The model under review builds one solid part; all positions refer to its coordinate system, in mm. Face numbers are marked on the shaded views. Round coordinates to 2 decimals unless told otherwise and drop trailing zeros. Write each loop counter-clockwise with the first axis right and the second up, starting at its lowest first coordinate (ties: lowest second). Pieces come first, ordered by that corner, then holes.
Item 1: Add section B-B (x = 0). Give the boundary of the cut face in (y, z).
Item 2: Add section A-A (y = 3.75). Give the boundary of the cut face in (x, z), plus the area to 3 significant figures.
Item 3: Clearance check with flat-ended pins moving along their axes: pin 1 Ø3 at (y, z) = (15.5, -5) entering from +X; pin 2 Ø8 at (y, z) = (9, 7.5) entering from -X; pin 3 Ø4 at (x, y) = (13, 3.5) entering from -Z; pin 4 Ø18 at (x, z) = (0, 0) entering from +Y. State where each tip first meets the part, or that it passes through.
Item 4: To check wall thickness, follow L1, parallel to Z at x = 0, y = 7.5; L2, parallel to X at y = 8.5, z = 0; L3, parallel to X at y = 1.25, z = -4. State the ranges of each line that lie inside material, in increasing order.
Item 5: Draft analysis for pull direction Z (two halves, no side actions). For the marked faces 1, 2 and 3, state which applies: +Z half, -Z half, draft (parallel to the pull), parting line (faces both ways), or undercut.
```python
from build123d import *

# Parameters (mm, degrees)
SKETCH5_R           = 10
BOSS_EXTRUDE1_DEPTH = 20


with BuildPart() as part:
    # Sketch5 → Boss-Extrude1 (new body)
    with BuildSketch(Plane(origin=(0, 0, 0), x_dir=(1, 0, 0), z_dir=(0, 1, 0))):
        Polygon((19.976319314, 0), (9.988159657, 17.3), (-9.988159657, 17.3), (-19.976319314, 0), (-9.988159657, -17.3), (9.988159657, -17.3), align=None)
        Circle(SKETCH5_R, mode=Mode.SUBTRACT)
    extrude(amount=BOSS_EXTRUDE1_DEPTH)

    # Sketch6 → Cut-Revolve1 (revolve, cut)
    with BuildSketch(Plane.XY):
        Polygon((19.976319314, 0), (16.976319314, 0), (19.976319314, 3), align=None)
        Polygon((19.976319314, 20), (16.976319314, 20), (19.976319314, 17), align=None)
    revolve(axis=Axis((0, 0, 0), (0, 1, 0)), mode=Mode.SUBTRACT)


solid = part.part
```
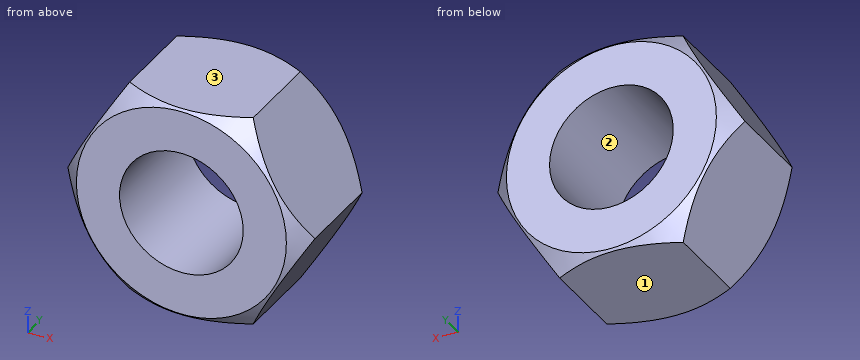
Numbers:
1. outline: (0, -16.98) - (0.32, -17.3) - (19.68, -17.3) - (20, -16.98) - (20, -10) - (0, -10) - close; (0, 10) - (20, 10) - (20, 16.98) - (19.68, 17.3) - (0.32, 17.3) - (0, 16.98) - close
2. outline: (-19.98, 0) - (-9.99, -17.3) - (9.99, -17.3) - (19.98, 0) - (9.99, 17.3) - (-9.99, 17.3) - close; hole circle Ø20 at (0, 0)
2. area: 723 mm2
3. pin 1: stops at x = 17.96
3. pin 2: stops at x = -17.96
3. pin 3: stops at z = -15.55
3. pin 4: passes through
4. L1: z = -17.3 to -10, 10 to 17.3
4. L2: x = -19.98 to -10, 10 to 19.98
4. L3: x = -17.67 to -9.17, 9.17 to 17.67
5. face 1: -Z half
5. face 2: undercut
5. face 3: +Z half
